Print and shaded views of the part. All mm, measured from the part's lowest x, y and z. A direction names the side the tool comes from. Round coordinates to 2 decimals unless told otherwise and drop trailing zeros. Write each loop counter-clockwise with the first axis right and the second up, starting at its lowest first coordinate (ties: lowest second). Pieces come first, ordered by that corner, then holes. Notation, with made-up numbers: (-38.75, -5.75) - (11.25, -5.75) arc R25 ccw to (11.25, 6.25) - close; hole circle Ø6 at (56, 71). An arc over 180 degrees is marked (long way). Put each result on its own line as item: value. Start each with the question number.
Item 1: Pin check, flat tip, straight feed: pin 1 Ø4 at (x, z) = (15, 40) entering from -Y. Stop position of the tip, or through.
Item 2: Cut at A-A (y = 25). Give the cut face in (x, z), and give its area (3 significant figures).
Item 3: Cut at C-C (x = 15.75). Give the cut face in (y, z).
Item 4: 3-axis set-ups, long thin cutter, end or side, ignore diameter. For the marked faces 1 and 2: which of +Z, -Z, +X, -X, +Y, -Y reach the whole face in a straight line?
Item 5: Drill centre lines: line 1 (Z direction, x = 1.2, y = 25); line 2 (Y direction, x = 27.2, z = 40); line 3 (X direction, y = 26, z = 50.5). Where is each one in solid material? Low to high. Write a range as from..to.
Item 6: Cut at B-B (z = 40). Give the cut face in (x, y).
Item 7: Cut at D-D (z = 50.5). Give the cut face in (x, y), and give its area (3 significant figures).
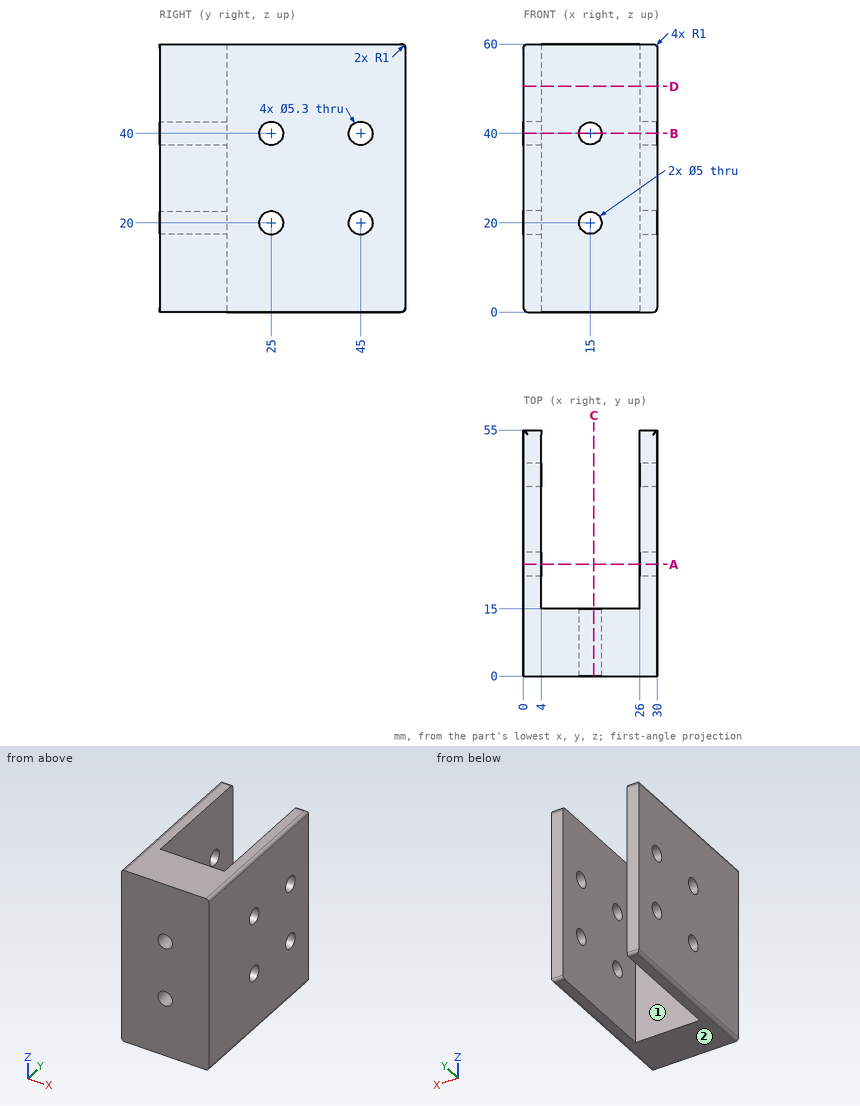
Output values:
1. pin 1: through
2. outline: (0, 1) arc R1 ccw to (1, 0) - (4, 0) - (4, 17.35) - (0, 17.35) - close; (0, 22.65) - (4, 22.65) - (4, 37.35) - (0, 37.35) - close; (0, 42.65) - (4, 42.65) - (4, 60) - (1, 60) arc R1 ccw to (0, 59) - close; (26, 0) - (29, 0) arc R1 ccw to (30, 1) - (30, 17.35) - (26, 17.35) - close; (26, 22.65) - (30, 22.65) - (30, 37.35) - (26, 37.35) - close; (26, 42.65) - (30, 42.65) - (30, 59) arc R1 ccw to (29, 60) - (26, 60) - close
2. area: 394 mm2
3. outline: (0, 0) - (15, 0) - (15, 17.62) - (0, 17.62) - close; (0, 22.38) - (15, 22.38) - (15, 37.62) - (0, 37.62) - close; (0, 42.38) - (15, 42.38) - (15, 60) - (0, 60) - close
4. face 1: +Z, -Z, +Y
4. face 2: -Z, +X, -X, +Y, -Y
5. line 1: 0..17.35, 22.65..37.35, 42.65..60
5. line 2: 0..22.35, 27.65..42.35, 47.65..55
5. line 3: 0..4, 26..30
6. outline: (0, 0) - (12.5, 0) - (12.5, 15) - (4, 15) - (4, 22.35) - (0, 22.35) - close; (0, 27.65) - (4, 27.65) - (4, 42.35) - (0, 42.35) - close; (0, 47.65) - (4, 47.65) - (4, 55) - (0, 55) - close; (17.5, 0) - (30, 0) - (30, 22.35) - (26, 22.35) - (26, 15) - (17.5, 15) - close; (26, 27.65) - (30, 27.65) - (30, 42.35) - (26, 42.35) - close; (26, 47.65) - (30, 47.65) - (30, 55) - (26, 55) - close
7. outline: (0, 0) - (30, 0) - (30, 55) - (26, 55) - (26, 15) - (4, 15) - (4, 55) - (0, 55) - close
7. area: 770 mm2
